Check sheet for the drawn part. Datum: minimum x, y, z corner. Units: mm. A direction names the side the tool comes from. Coordinates: 2 decimals unless noted, no trailing zeros. Order: outer loops, then holes, each group sorted by start corner. A loop starts at its lowest first (then second) coordinate and runs counter-clockwise, first axis right, second up. Notation, with made-up numbers: (-11, 89) - (26, 89) arc R22 ccw to (26, 101) - close; hole circle Ø4 at (41, 74.25). An arc over 180 degrees is marked (long way). Return JSON: item names as keys, results as strings. Group by question number.
Item 1: Section check A-A on x = 19.25. Enter the section's corners in (y, z), then the cut area to 3 significant figures.
Item 2: Scan lines: probe 1 along X at (y, z) = (100, 43); probe 2 along Y at (x, z) = (20, 17); probe 3 along Y at (x, z) = (10.75, 35.5). Record each from-to range of solid material in increasing order.
Item 3: Section check B-B on y = 100. Enter the section's corners in (x, z), then the cut area to 3 significant figures.
Item 4: Section check D-D on x = 10.75. Enter the section's corners in (y, z), then the cut area to 3 significant figures.
Item 5: Section check C-C on z = 13. Enter the section's corners in (x, y).
Item 6: Gauge pin test, flat ends, axial feed: pin 1 (3 mm diameter, centred on x = 9, y = 18, fed in from +Z); pin 2 (6 mm diameter, centred on x = 8, z = 7, fed in from +Y); pin 3 (5 mm diameter, centred on x = 4.5, y = 68.5, fed in from -Z). Record the tip position at first contact, or that the pin passes through.
Item 7: Tool access check on the marked faces 1, 2 and 3. Record the directions out of +Z, -Z, +X, -X, +Y, -Y that give a thin tool (end or side, any length) a straight path to the whole face; none if there is none.
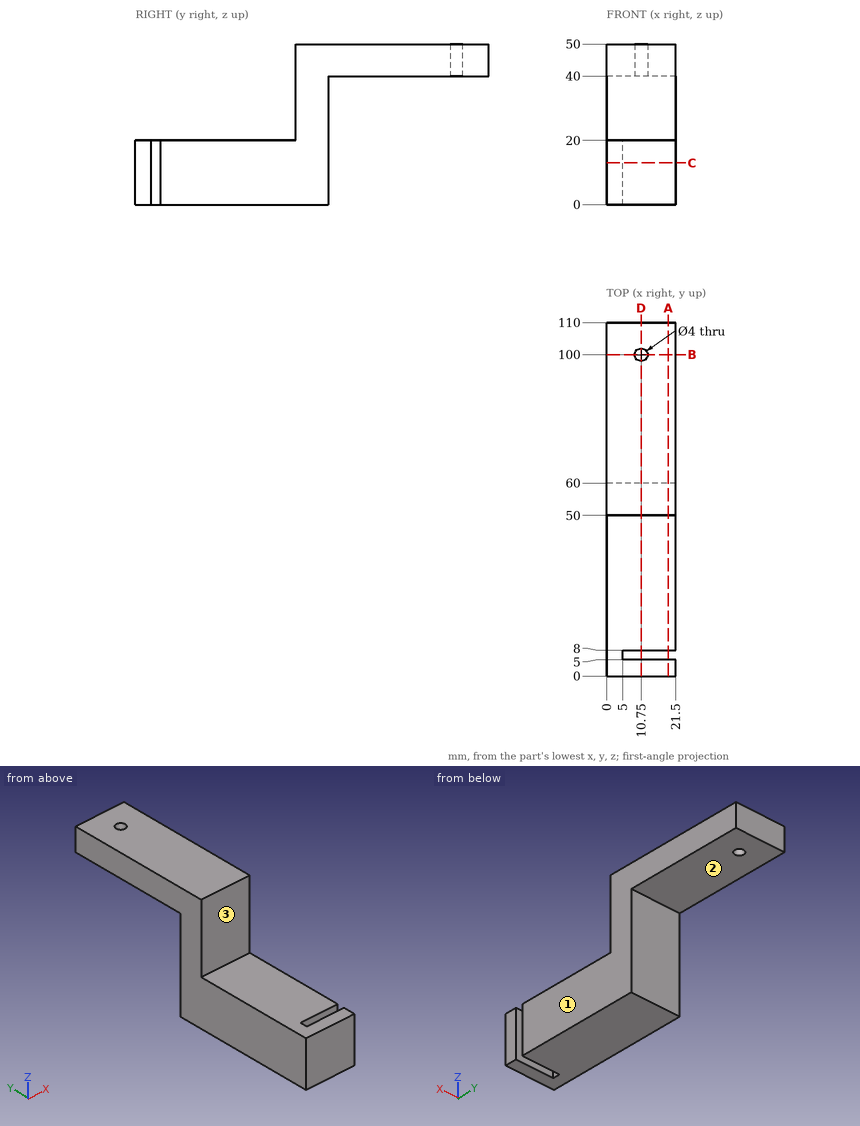
Computed:
{
 "1": {"outline": "(0, 0) - (5, 0) - (5, 20) - (0, 20) - close; (8, 0) - (60, 0) - (60, 40) - (110, 40) - (110, 50) - (50, 50) - (50, 20) - (8, 20) - close", "area": "1,940 mm²"},
 "2": {"probe 1": "x = 0 to 8.75, 12.75 to 21.5", "probe 2": "y = 0 to 5, 8 to 60", "probe 3": "y = 50 to 60"},
 "3": {"outline": "(0, 40) - (8.75, 40) - (8.75, 50) - (0, 50) - close; (12.75, 40) - (21.5, 40) - (21.5, 50) - (12.75, 50) - close", "area": "175 mm²"},
 "4": {"outline": "(0, 0) - (5, 0) - (5, 20) - (0, 20) - close; (8, 0) - (60, 0) - (60, 40) - (98, 40) - (98, 50) - (50, 50) - (50, 20) - (8, 20) - close; (102, 40) - (110, 40) - (110, 50) - (102, 50) - close", "area": "1,900 mm²"},
 "5": {"outline": "(0, 0) - (21.5, 0) - (21.5, 5) - (5, 5) - (5, 8) - (21.5, 8) - (21.5, 60) - (0, 60) - close"},
 "6": {"pin 1": "stops at z = 20", "pin 2": "stops at y = 60", "pin 3": "stops at z = 40"},
 "7": {"face 1": "+Z, -Z, +X, +Y, -Y", "face 2": "-Z, +X, -X, +Y", "face 3": "+Z, +X, -X, -Y"}
}
